from build123d import *

# Parameters (mm, degrees)
SKETCH1_W           = 10.62
SKETCH1_H           = 6.3
BOSS_EXTRUDE1_DEPTH = 8.8
SKETCH2_W           = 0.8
SKETCH2_H           = 0.5
BOSS_EXTRUDE2_DEPTH = 3.6
CUT_EXTRUDE1_REACH  = 12.62
SKETCH4_W           = 2
SKETCH4_H           = 4
CUT_EXTRUDE2_DEPTH  = 3.15
CUT_EXTRUDE2_TAPER  = 10


with BuildPart() as part:
    # Sketch1 → Boss-Extrude1 (new body)
    with BuildSketch(Plane(origin=(0, 0, 0), x_dir=(1, 0, 0), z_dir=(0, 1, 0))):
        Rectangle(SKETCH1_W, SKETCH1_H)
    extrude(amount=BOSS_EXTRUDE1_DEPTH)

    # Sketch2 → Boss-Extrude2 (add)
    with BuildSketch(Plane(origin=(0, 0, 0), x_dir=(1, 0, 0), z_dir=(0, 1, 0))):
        with Locations((1.27, 0.2)):
            Rectangle(SKETCH2_W, SKETCH2_H)
        with Locations((3.81, 0.2)):
            Rectangle(SKETCH2_W, SKETCH2_H)
        with Locations((-1.27, 0.2)):
            Rectangle(SKETCH2_W, SKETCH2_H)
        with Locations((-3.81, 0.2)):
            Rectangle(SKETCH2_W, SKETCH2_H)
    extrude(amount=-BOSS_EXTRUDE2_DEPTH)

    # Sketch3 → Cut-Extrude1 (cut, up to next)
    with BuildSketch(Plane(origin=(5.31, 0, 0), x_dir=(0, 0, -1), z_dir=(1, 0, 0)), mode=Mode.PRIVATE) as cut_extrude1_sk1:
        with BuildLine():
            ThreePointArc((-3.15, 4.7), (-2.974264069, 5.124264069), (-2.55, 5.3))
            Line((-2.55, 5.3), (-2.337822174, 5.3))
            Line((-2.337822174, 5.3), (-1.4, 8.8))
            Line((-1.4, 8.8), (-3.15, 8.8))
            Line((-3.15, 8.8), (-3.15, 4.7))
        make_face()
    cut_extrude1_tool1 = extrude(cut_extrude1_sk1.sketch, amount=-CUT_EXTRUDE1_REACH, mode=Mode.PRIVATE) & part.part
    add(cut_extrude1_tool1.solids().sort_by_distance((5.31, 7.227986, 2.489914))[0], mode=Mode.SUBTRACT)
    # Sketch3 → Cut-Extrude1 (cut, up to next)
    with BuildSketch(Plane(origin=(5.31, 0, 0), x_dir=(0, 0, -1), z_dir=(1, 0, 0)), mode=Mode.PRIVATE) as cut_extrude1_sk2:
        Polygon((3.15, 8.8), (1.4, 8.8), (3.15, 2.268911087), align=None)
    cut_extrude1_tool2 = extrude(cut_extrude1_sk2.sketch, amount=-CUT_EXTRUDE1_REACH, mode=Mode.PRIVATE) & part.part
    add(cut_extrude1_tool2.solids().sort_by_distance((5.31, 6.62297, -2.566667))[0], mode=Mode.SUBTRACT)

    # Sketch4 → Cut-Extrude2 (cut)
    with BuildSketch(Plane.XY.offset(3.15)):
        with Locations((-3.81, 2.268911087)):
            Rectangle(SKETCH4_W, SKETCH4_H)
        with Locations((-1.27, 2.268911087)):
            Rectangle(SKETCH4_W, SKETCH4_H)
        with Locations((1.27, 2.268911087)):
            Rectangle(SKETCH4_W, SKETCH4_H)
        with Locations((3.81, 2.268911087)):
            Rectangle(SKETCH4_W, SKETCH4_H)
    extrude(amount=-CUT_EXTRUDE2_DEPTH, taper=CUT_EXTRUDE2_TAPER, mode=Mode.SUBTRACT)


solid = part.part
Model file for the job. Use its own axes, mm. A direction names the side the tool comes from. Give positions to 0.01 mm unless a question says otherwise; leave off trailing zeros. Loops run counter-clockwise (first coordinate to the right, second up) from the corner with the lowest first, then second, coordinate; pieces in that order, holes last.
1) Pull direction Y, two halves, no side cores. Call faces 3 (the flat face through (0.074, 5.58, -2.263)), 4 (the flat face through (1, 2, 0)), 5 (the flat face through (0, 1, -3.15)): +Y half, -Y half, draft (parallel to the pull), parting line (faces both ways), or undercut.
2) Wall check: line 1 (X direction, y = -1, z = 0); line 2 (X direction, y = 2, z = 0.25); line 3 (X direction, y = 2.5, z = 0.5). Give the ranges that are in metal, low to high.
3) Flat gauge pins, fed straight in: pin 1 Ø0.6 at (y, z) = (-2.5, 0) entering from +X; pin 2 Ø1 at (x, y) = (1, 5.5) entering from -Z; pin 3 Ø0.6 at (x, y) = (3.5, -1) entering from +Z. Where does each tip first touch, or does it go through?
4) Saw through at C-C (z = 2.75). Count the separate pieces of the cut face and the enclosed holes in it, plus the area to 3 significant figures.
5) Saw through at B-B (z = -1.25). Write the cut outline in (x, y).
6) Saw through at D-D (y = 7.75). Write the cut outline in (x, z), plus the area to 3 significant figures.
7) Tool access for faces 1 (the flat face through (-4, 2, 0)), 2 (the flat face through (0, 2, 3.15)): list every direction of +Z, -Z, +X, -X, +Y, -Y with a clear straight run to the whole face (end or side of a thin tool).
8) Saw through at A-A (y = -1.75). Write the cut outline in (x, z).
Answer block:
1. face 3: +Y half
1. face 4: undercut
1. face 5: draft
2. line 1: x = -4.21 to -3.41, -1.67 to -0.87, 0.87 to 1.67, 3.41 to 4.21
2. line 2: x = -5.31 to -4.3, -3.32 to -1.76, -0.78 to 0.78, 1.76 to 3.32, 4.3 to 5.31
2. line 3: x = -5.31 to -4.34, -3.28 to -1.8, -0.74 to 0.74, 1.8 to 3.28, 4.34 to 5.31
3. pin 1: stops at x = 4.21
3. pin 2: stops at z = -2.42
3. pin 3: stops at z = 0.05
4. separate pieces: 1
4. enclosed holes: 4
4. area: 27.2 mm2
5. outline: (-5.31, 0) - (5.31, 0) - (5.31, 8.8) - (-5.31, 8.8) - close
6. outline: (-5.31, -1.68) - (5.31, -1.68) - (5.31, 1.68) - (-5.31, 1.68) - close
6. area: 35.7 mm2
7. face 1: +Z
7. face 2: +Z, +X, -X, +Y, -Y
8. outline: (-4.21, -0.45) - (-3.41, -0.45) - (-3.41, 0.05) - (-4.21, 0.05) - close; (-1.67, -0.45) - (-0.87, -0.45) - (-0.87, 0.05) - (-1.67, 0.05) - close; (0.87, -0.45) - (1.67, -0.45) - (1.67, 0.05) - (0.87, 0.05) - close; (3.41, -0.45) - (4.21, -0.45) - (4.21, 0.05) - (3.41, 0.05) - close
